For this review, use the dimensioned drawing (mm, ordinates from the lowest corner) and the shaded views. A direction names the side the tool comes from. Round coordinates to 2 decimals unless told otherwise and drop trailing zeros. Order: outer loops, then holes, each group sorted by start corner. A loop starts at its lowest first (then second) coordinate and runs counter-clockwise, first axis right, second up. Notation, with made-up numbers: (48.25, 18.5) - (54.25, 18.5) arc R17 cw to (54.25, 30.5) - close; hole circle Ø8 at (8, 89.25). An arc over 180 degrees is marked (long way). Write item = value, one per line.
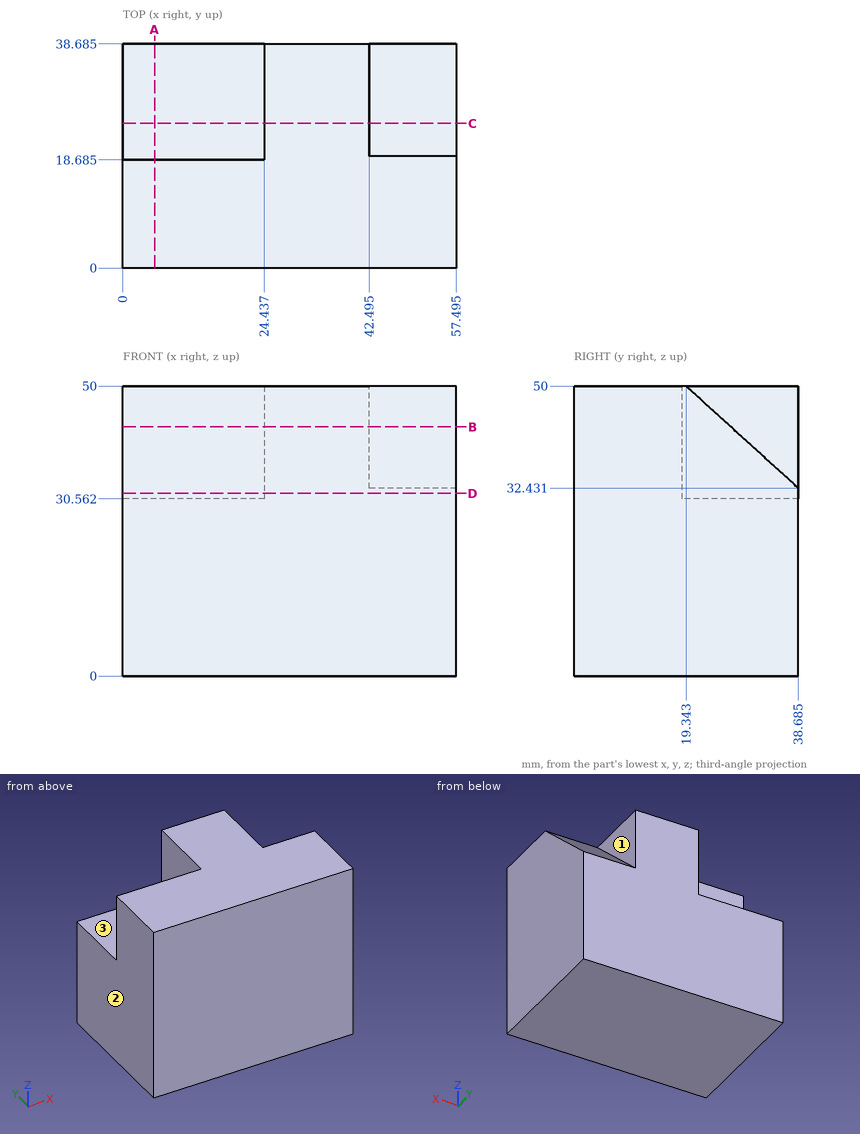
Item 1: Take a section at B-B, the plane z = 43. State the section outline as (x, y) points (1 decimal).
Data:
outline = (0, 0) - (57.5, 0) - (57.5, 27) - (42.5, 27) - (42.5, 38.7) - (24.4, 38.7) - (24.4, 18.7) - (0, 18.7) - close
Item 2: Take a section at C-C, the plane y = 25. State the section outline as (x, z) points (1 decimal).
Data:
outline = (0, 0) - (57.5, 0) - (57.5, 44.9) - (42.5, 44.9) - (42.5, 50) - (24.4, 50) - (24.4, 30.6) - (0, 30.6) - close
Item 3: Take a section at A-A, the plane x = 5.5. State the section outline as (y, z) points (1 decimal).
Data:
outline = (0, 0) - (38.7, 0) - (38.7, 30.6) - (18.7, 30.6) - (18.7, 50) - (0, 50) - close
Item 4: Insertion check: P1, Ø15.5, axis at y = 33, z = 39.5, coming from the -X side; P2, Ø9.5, axis at x = 14.5, z = 40.5, coming from the +Y side (1 decimal). Each pin has a flat end and moves straight along its axis. Give the tip position at first contact, or say it passes through.
Data:
P1 = 24.44
P2 = 18.7
Item 5: For line 1 along Z through (x, y) = (3, 31.5); line 2 along X through (y, z) = (22, 40.5) (1 decimal); line 3 along Y through (x, z) = (3, 44) (1 decimal), list the stretches that pass through material, from the lowest coordinate up. Write a range as [from, to].
Data:
line_1 = [0, 30.56]
line_2 = [24.4, 57.5]
line_3 = [0, 18.7]
Item 6: Take a section at D-D, the plane z = 31.5. State the section outline as (x, y) points (1 decimal).
Data:
outline = (0, 0) - (57.5, 0) - (57.5, 38.7) - (24.4, 38.7) - (24.4, 18.7) - (0, 18.7) - close
Item 7: For the marked faces 1, 2 and 3, list the 3-axis set-ups (+Z, -Z, +X, -X, +Y, -Y) from which the entire face can be reached by the end or side of a thin tool; tool diameter is ignored.
Data:
face_1 = +Z, +X, +Y
face_2 = +Z, -Z, -X, +Y, -Y
face_3 = +Z, -X, +Y
